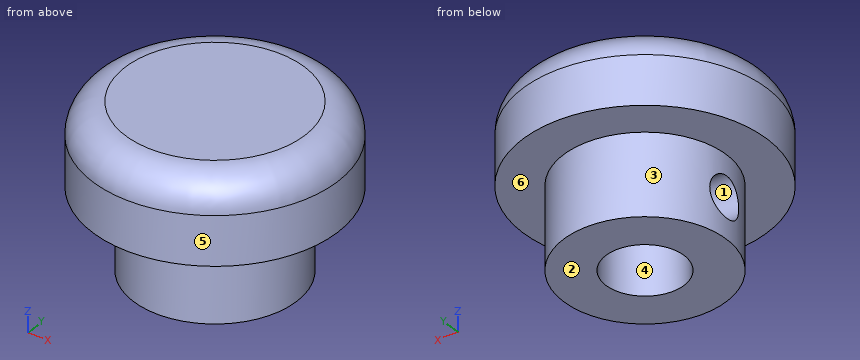
Autodesk Inventor part; units mm, degrees
ref_plane "YZ Plane" through (0, 0, 0) normal (1, 0, 0) x (0, 1, 0)
ref_plane "XZ Plane" through (0, 0, 0) normal (0, 1, 0) x (-1, 0, 0)
ref_plane "XY Plane" through (0, 0, 0) normal (0, 0, 1) x (1, 0, 0)
sketch "Sketch1" plane through (0, 0, 0) normal (0, 0, 1) x (1, 0, 0)
  circle A0 centre (0, 0) radius 2.4
  circle A1 centre (0, 0) radius 5
  dimension "d0" = 4.8
  dimension "d1" = 10
extrude "Extrusion1" add sketch "Sketch1" along normal blind 5
sketch "Sketch2" plane through (0, 0, 5) normal (0, 0, 1) x (1, 0, 0)
  circle A0 centre (0, 0) radius 7.5
  dimension "d4" = 15
extrude "Extrusion2" add sketch "Sketch2" along normal blind 5
fillet "Fillet1" radius 2 1 edges at (-7.5, 0, 10)
sketch "Sketch3" plane through (0, 0, 0) normal (1, 0, 0) x (0, 1, 0)
  line L0 (5, 0) -> (-5, 0)
  point P0 (0, 0)
  point P1 (0, 2.5)
  dimension "d8" = 2.5
hole "Hole1" at (0, 0, 2.5) direction (-1, 0, 0) diameter 2.5 end through all
properties part number "10-03-011 Ciuperca"
The model under review builds one solid part; all positions refer to its coordinate system, in mm. Face numbers are marked on the shaded views. A direction names the side the tool comes from. Give positions to 0.01 mm unless a question says otherwise; leave off trailing zeros. Order: outer loops, then holes, each group sorted by start corner. A loop starts at its lowest first (then second) coordinate and runs counter-clockwise, first axis right, second up. Notation, with made-up numbers: M 48,-5.75 L 83,-5.75 A31 cw 83,28.25 Z; hole C -36.75,60 d11. An arc over 180 degrees is marked long. Answer in a Markdown table with one row per item. Add a question column.
1. Machinability: for the marked faces 1, 2 and 3, which of the approach directions +Z, -Z, +X, -X, +Y, -Y give a long, thin tool a straight path to every point of the face, cutting with its end or side? Answer none if there is none.
2. Mouldability with a two-part tool opening along Y and no side actions: class the marked faces 4, 5 and 6 as released by +Y, released by -Y, zero draft, split by the parting line, or undercut.
3. Add section C-C on z = 5.5. State the section outline as (x, y) points, plus the area to 3 significant figures.
4. Add section D-D on z = 2. State the section outline as (x, y) points, plus the area to 3 significant figures.
5. For pin 1 Ø2 at (y, z) = (0, 2.5) entering from +X; pin 2 Ø4 at (x, z) = (5.5, 7.5) entering from -Y; pin 3 Ø5 at (y, z) = (5, 4) entering from +X, all flat-tipped, find the tip position at first contact; note any pin that passes through.
6. To check wall thickness, follow line 1 along Y through (x, z) = (0, 3.1); line 2 along Y through (x, z) = (-2.5, 2.25). State the ranges of each line that lie inside material, in increasing order.
7. Add section A-A on y = 0. State the section outline as (x, z) points, plus the area to 3 significant figures.
8. Add section B-B on x = 0. State the section outline as (y, z) points, plus the area to 3 significant figures.
The answers:
| question | item | result |
|---|---|---|
| 1 | face 1 | -X |
| 1 | face 2 | -Z, +X, -X, +Y, -Y |
| 1 | face 3 | -Z |
| 2 | face 4 | undercut |
| 2 | face 5 | split by the parting line |
| 2 | face 6 | zero draft |
| 3 | outline | C 0,0 d15 |
| 3 | area | 177 mm2 |
| 4 | outline | M -4.87,-1.15 A5 ccw long -4.87,1.15 L -2.11,1.15 A2.4 cw long -2.11,-1.15 Z |
| 4 | area | 54.4 mm2 |
| 5 | pin 1 | x = 5 |
| 5 | pin 2 | y = -6.63 |
| 5 | pin 3 | x = 6.99 |
| 6 | line 1 | -5 to -2.4, 2.4 to 5 |
| 6 | line 2 | -4.33 to -1.22, 1.22 to 4.33 |
| 7 | outline | M -7.5,5 L -5,5 L -5,3.75 L -2.4,3.75 L -2.4,5 L 2.4,5 L 2.4,0 L 5,0 L 5,5 L 7.5,5 L 7.5,8 A2 ccw 5.5,10 L -5.5,10 A2 ccw -7.5,8 Z; M -5,0 L -2.4,0 L -2.4,1.25 L -5,1.25 Z |
| 7 | area | 92.8 mm2 |
| 8 | outline | M -7.5,5 L -5,5 L -5,0 L -2.4,0 L -2.4,5 L 2.4,5 L 2.4,0 L 5,0 L 5,5 L 7.5,5 L 7.5,8 A2 ccw 5.5,10 L -5.5,10 A2 ccw -7.5,8 Z |
| 8 | area | 99.3 mm2 |
